```python
from build123d import *

# Parameters (mm, degrees)
F0_W     = 40
F0_H     = 10
F1_DEPTH = 0.5
F2_W     = 10
F2_H     = 10
F3_DEPTH = 10
F4_W     = 10
F4_H     = 10
F4_W_2   = 30
F5_DEPTH = 1
F6_R     = 4.99999
F7_R     = 2.5
F8_DEPTH = 25
F9_SIZE  = 3


# Not quite as in the source:
# - a fillet or chamfer is up to 0.001 mm smaller than in the source, because OpenCascade refuses the exact size


with BuildPart() as f1:
    # F0 (on Top) → F1 (new body)
    with BuildSketch(Plane.XY):
        Rectangle(F0_W, F0_H)
    extrude(amount=F1_DEPTH)

    # F2 (on face) → F3 (join)
    with BuildSketch(Plane.XY.offset(0.5)):
        with Locations((-15, 0)):
            Rectangle(F2_W, F2_H)
        with Locations((15, 0)):
            Rectangle(F2_W, F2_H)
    extrude(amount=F3_DEPTH)

    # F4 (on face) → F5 (join)
    with BuildSketch(Plane.XY.offset(10.5)):
        with Locations((-15, 0)):
            Rectangle(F4_W, F4_H)
        with Locations((5, 0)):
            Rectangle(F4_W_2, F4_H)
    extrude(amount=F5_DEPTH)

    # F6 (radius 5 in the source; OpenCascade refuses exactly that, so slightly less here)
    f6_edges = [f1.edges().sort_by_distance(p)[0] for p in [
        (20, -5, 5.75),
        (20, 5, 5.75),
    ]]
    fillet(f6_edges, radius=F6_R)

    # F7 (on face) → F8 (cut)
    with BuildSketch(Plane.XY.offset(11.5)):
        with Locations((-15, 0)):
            Circle(F7_R)
    extrude(amount=-F8_DEPTH, mode=Mode.SUBTRACT)

    # F9
    f9_edges = [f1.edges().sort_by_distance(p)[0] for p in [
        (-20, 5, 5.75),
        (-10, 5, 5.5),
    ]]
    chamfer(f9_edges, length=F9_SIZE)


solid = f1.part
```
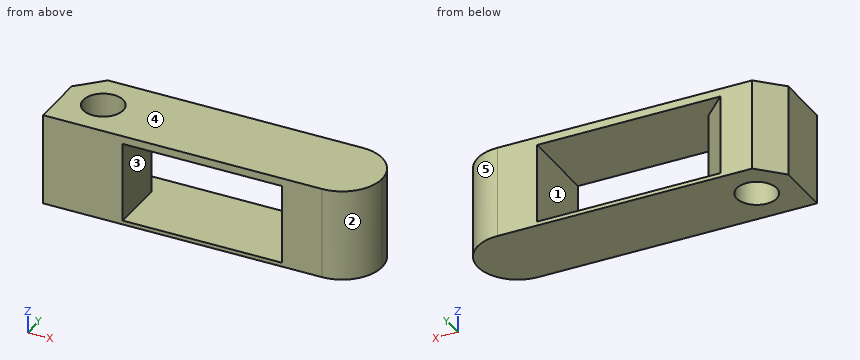
Source: CAD feature listing. Evaluate the final solid. Frame: model axes, mm. Face numbers are marked on the shaded views. A direction names the side the tool comes from. Give positions to 0.01 mm unless a question says otherwise; leave off trailing zeros. Write each loop counter-clockwise with the first axis right and the second up, starting at its lowest first coordinate (ties: lowest second). Pieces come first, ordered by that corner, then holes. Notation, with made-up numbers: (11.25, 33) - (29.25, 33) arc R17 ccw to (29.25, 64) - close; hole circle Ø9 at (15.25, 80.25). An arc over 180 degrees is marked (long way). One line per item, written item: value. Start each with the question number.
Q1. Material intervals for probe 1 along Z at (x, y) = (8, -3.75); probe 2 along X at (y, z) = (0.25, 9.75); probe 3 along X at (y, z) = (0.75, 5.75), sorted ascending. Write a range as from..to.
Q2. Section query B-B, the plane x = -8. Return the cut outline in (y, z).
Q3. Section query A-A, the plane z = 2.25. Count the separate pieces of the cut face and the enclosed holes in it, then the cut area to 3 significant figures.
Q4. Section query D-D, the plane x = -12. Return the cut outline in (y, z).
Q5. First-contact query: pin 1 Ø1.5 at (x, z) = (7.5, 4) entering from -Y. Flat tip, straight axial feed; report the tip coordinate or a pass-through.
Q6. Section query C-C, the plane y = -4. Return the cut outline in (x, z), then the cut area to 3 significant figures.
Q7. Draft query along Z for the marked faces 3, 4 and 5. Return one class per face: +Z half, -Z half, draft (parallel to the pull), parting line (faces both ways), or undercut.
Q8. Set-up query: the marked faces 1 and 2. Return all of +Z, -Z, +X, -X, +Y, -Y with unobstructed straight access to the full face (end or side cutting, diameter ignored); none if empty.
Answer:
1. probe 1: z = 0..0.5, 10.5..11.5
1. probe 2: x = -20..-17.49, -12.51..-10, 10..19.99
1. probe 3: x = -20..-17.38, -12.62..-10, 10..19.94
2. outline: (-5, 0) - (5, 0) - (5, 0.5) - (-5, 0.5) - close; (-5, 10.5) - (5, 10.5) - (5, 11.5) - (-5, 11.5) - close
3. separate pieces: 2
3. enclosed holes: 1
3. area: 161 mm2
4. outline: (-5, 0) - (5, 0) - (5, 0.5) - (4, 0.5) - (4, 10.5) - (5, 10.5) - (5, 11.5) - (-5, 11.5) - close
5. pin 1: passes through
6. outline: (-20, 0) - (18, 0) - (18, 11.5) - (-20, 11.5) - close; hole (-10, 0.5) - (10, 0.5) - (10, 10.5) - (-10, 10.5) - close
6. area: 237 mm2
7. face 3: undercut
7. face 4: +Z half
7. face 5: draft
8. face 1: +Y, -Y
8. face 2: +Z, -Z, +X, -Y
